The drawing under review shows one solid part. Ordinate dimensions are in mm from its lowest x, y, z. Coordinates: 2 decimals unless noted, no trailing zeros. Loops run counter-clockwise (first coordinate to the right, second up) from the corner with the lowest first, then second, coordinate; pieces in that order, holes last. Notation, with made-up numbers: (23.25, 43.25) -> (39.25, 43.25) arc R18 cw to (39.25, 78.25) -> close; hole circle Ø4 at (-9, 43). An arc over 180 degrees is marked (long way). Use a Markdown table: item, result.
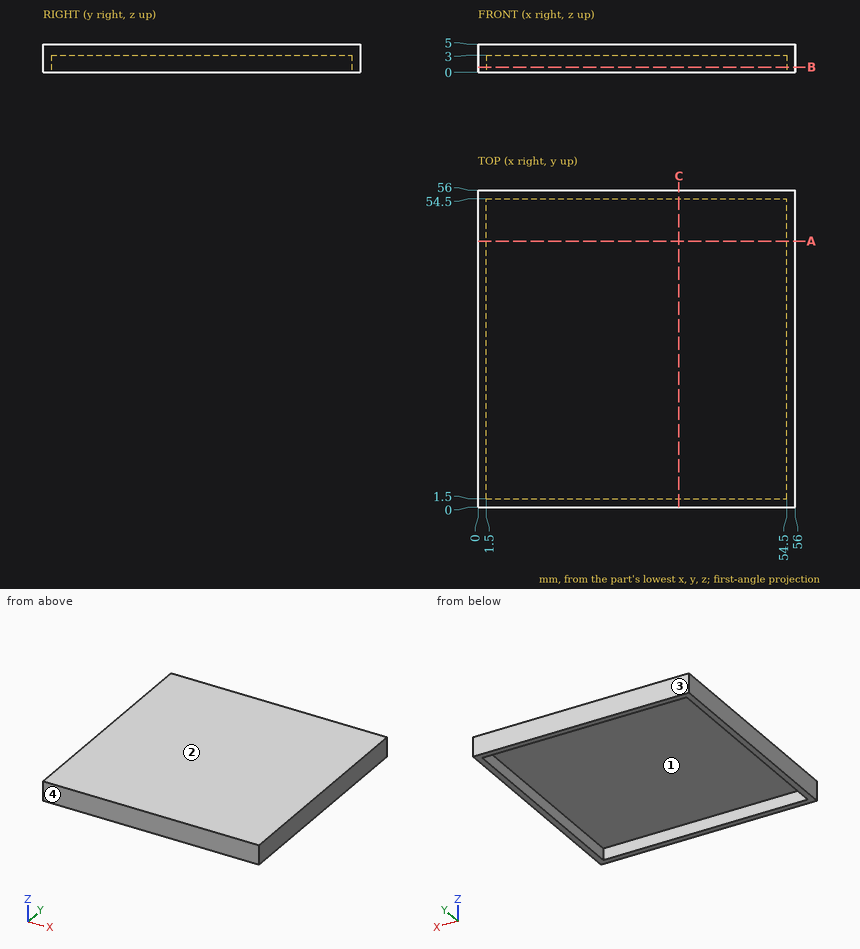
(1) Take a section at B-B on z = 0.9. Write out the cut boundary in (x, y), plus the area to 3 significant figures.
Found:
| item | result |
|---|---|
| outline | (0, 0) -> (56, 0) -> (56, 56) -> (0, 56) -> close; hole (1.5, 1.5) -> (54.5, 1.5) -> (54.5, 54.5) -> (1.5, 54.5) -> close |
| area | 327 mm^2 |
(2) Take a section at A-A on y = 47. Write out the cut boundary in (x, z), plus the area to 3 significant figures.
Found:
| item | result |
|---|---|
| outline | (0, 0) -> (1.5, 0) -> (1.5, 3) -> (54.5, 3) -> (54.5, 0) -> (56, 0) -> (56, 5) -> (0, 5) -> close |
| area | 121 mm^2 |
(3) Mouldability with a two-part tool opening along Y and no side actions: class the marked faces 1, 2, 3 and 4 as pulls with the +Y half, pulls with the -Y half, needs draft (parallel to the pull), parting line crosses it, or undercut.
Found:
| item | result |
|---|---|
| face 1 | undercut |
| face 2 | needs draft |
| face 3 | pulls with the +Y half |
| face 4 | pulls with the -Y half |
(4) For line 1 along Y through (x, z) = (47, 2.9); line 2 along Z through (x, y) = (46, 51), list the stretches that pass through material, from the lowest coordinate up.
Found:
| item | result |
|---|---|
| line 1 | y = 0 to 1.5, 54.5 to 56 |
| line 2 | z = 3 to 5 |
